Geometry: final body of the model. Coordinates: model frame, mm. A direction names the side the tool comes from. Round coordinates to 2 decimals unless told otherwise and drop trailing zeros. Order: outer loops, then holes, each group sorted by start corner. A loop starts at its lowest first (then second) coordinate and runs counter-clockwise, first axis right, second up. Notation, with made-up numbers: M 29.25,-10 L 40.25,-10 A15 ccw 40.25,13 Z; hole C 33.5,12.25 d5. An arc over 180 degrees is marked long. Return JSON: item names as keys, results as strings. Group by question number.
Q1. Contact query for flat-ended pins moving along their axis: pin 1 (1 mm diameter, centred on x = 7, y = 5.5, fed in from +Z); pin 2 (8 mm diameter, centred on y = 7, z = -21.5, fed in from +X); pin 3 (1.5 mm diameter, centred on y = 5, z = -22.5, fed in from +X). Output: stop coordinate, or through.
Q2. Cut plane B-B on x = -27.5. Output: boundary loops of the cut face in (y, z), and give its area (3 significant figures).
Q3. Cut plane C-C on z = 10.5. Output: boundary loops of the cut face in (x, y).
Q4. Ray query, probe 1 along X at (y, z) = (10, -0.5); probe 2 along Z at (x, y) = (20, 7.25); probe 3 along Z at (x, y) = (27, 2.5). Return the intervals inside material, ascending.
Q5. Access query for faces 5 (the face through (-1.99, 7.4, 32.71)), 6 (the face through (-13, 15, 30.5)). Directions: +Z, -Z, +X, -X, +Y, -Y. A direction counts if a zero-diameter tool reaches every point of the face in a straight line with its end or side. Return the directions, or none.
Q6. Mould query, pull axis Z, two halves, no side actions, for faces 1 (the face through (-0.079, 7.395, 33.052)), 2 (the face through (-13, 0, 30.5)), 3 (the face through (0, 7.4, -31.5)), 4 (the face through (1.96, 7.4, 32.7)). Classes: released by +Z, released by -Z, zero draft, split by the parting line, or undercut.
```python
from build123d import *

# Parameters (mm, degrees)
BOSS_EXTRUDE1_DEPTH = 15
CUT_EXTRUDE2_DEPTH  = 52.002935676


with BuildPart() as part:
    # Sketch1 → Boss-Extrude1 (new body)
    with BuildSketch(Plane(origin=(0, 0, 0), x_dir=(1, 0, 0), z_dir=(0, 1, 0))):
        with BuildLine():
            ThreePointArc((1.388184439, -34.024526654), (1.582903075, -34.267692689), (1.883792339, -34.348381715))
            ThreePointArc((1.883792339, -34.348381715), (24.448065102, -24.200250262), (34.365790759, -1.53376189))
            ThreePointArc((34.365790759, -1.53376189), (25.706615752, 22.858913066), (2.493104989, 34.309538433))
            ThreePointArc((2.493104989, 34.309538433), (1.837317334, 34.124415112), (1.452378604, 33.562142698))
            ThreePointArc((1.452378604, 33.562142698), (-0.029391592, 32.437392534), (-1.46595483, 33.619336656))
            ThreePointArc((-1.46595483, 33.619336656), (-1.844328043, 34.20829277), (-2.516198277, 34.404827707))
            ThreePointArc((-2.516198277, 34.404827707), (-25.784489967, 22.916882433), (-34.462378171, -1.538802818))
            ThreePointArc((-34.462378171, -1.538802818), (-24.537991164, -24.246863982), (-1.949992086, -34.441558533))
            ThreePointArc((-1.949992086, -34.441558533), (-1.638342507, -34.354295246), (-1.445420769, -34.094446164))
            ThreePointArc((-1.445420769, -34.094446164), (-0.053498551, -33.05116711), (1.388184439, -34.024526654))
        make_face()
        with BuildLine():
            Line((-2.417, 3.18717916), (0, 3.18717916))
            Line((0, 3.18717916), (2.417, 3.18717916))
            ThreePointArc((2.417, 3.18717916), (0, -4), (-2.417, 3.18717916))
        make_face(mode=Mode.SUBTRACT)
    extrude(amount=BOSS_EXTRUDE1_DEPTH)

    # Sketch2 → Cut-Extrude2 (cut, through all)
    with BuildSketch(Plane(origin=(0, 0, 0), x_dir=(1, 0, 0), z_dir=(0, 1, 0))):
        with BuildLine():
            ThreePointArc((-32.866935484, -2.96049859), (-23.334523779, -23.334523779), (-2.96049859, -32.866935484))
            ThreePointArc((-2.96049859, -32.866935484), (-1.9760642, -32.705835472), (-1.191889043, -32.089285714))
            ThreePointArc((-1.191889043, -32.089285714), (0, -31.5), (1.191889043, -32.089285714))
            ThreePointArc((1.191889043, -32.089285714), (1.9760642, -32.705835472), (2.96049859, -32.866935484))
            ThreePointArc((2.96049859, -32.866935484), (23.334523779, -23.334523779), (32.866935484, -2.96049859))
            ThreePointArc((32.866935484, -2.96049859), (25.333821586, 21.147044329), (2.96049859, 32.866935484))
            ThreePointArc((2.96049859, 32.866935484), (1.9760642, 32.705835472), (1.191889043, 32.089285714))
            ThreePointArc((1.191889043, 32.089285714), (0, 31.5), (-1.191889043, 32.089285714))
            ThreePointArc((-1.191889043, 32.089285714), (-1.9760642, 32.705835472), (-2.96049859, 32.866935484))
            ThreePointArc((-2.96049859, 32.866935484), (-25.333821586, 21.147044329), (-32.866935484, -2.96049859))
        make_face()
    extrude(amount=CUT_EXTRUDE2_DEPTH, mode=Mode.SUBTRACT)


solid = part.part
```
Result sheet:
{
 "1": {"pin 1": "stops at z = 33.78", "pin 2": "stops at x = 29.62", "pin 3": "stops at x = 26.65"},
 "2": {"outline": "M 0,-20.83 L 15,-20.83 L 15,-18.24 L 0,-18.24 Z; M 0,18.24 L 15,18.24 L 15,20.83 L 0,20.83 Z", "area": "77.6 mm²"},
 "3": {"outline": "M -32.86,0 L -31.28,0 L -31.28,15 L -32.86,15 Z; M 31.28,0 L 32.76,0 L 32.76,15 L 31.28,15 Z"},
 "4": {"probe 1": "x = -34.49 to -33, 33 to 34.4", "probe 2": "z = -27.99 to -26.25, 26.25 to 27.99", "probe 3": "z = -21.32 to -18.97, 18.97 to 21.32"},
 "5": {"face 5": "+Y, -Y", "face 6": "+Z, -Z, +X, -X, +Y"},
 "6": {"face 1": "released by +Z", "face 2": "zero draft", "face 3": "undercut", "face 4": "undercut"}
}
